from build123d import *

# Parameters (mm, degrees)
F0_W     = 210
F0_H     = 60
F1_DEPTH = 90
F2_T     = -2.5
F3_W     = 210
F3_H     = 60
F3_W_2   = 205
F3_H_2   = 55
F4_DEPTH = 2.5
F5_W     = 60
F5_H     = 50
F6_DEPTH = 25


with BuildPart() as f1:
    # F0 (on Top) → F1 (new body)
    with BuildSketch(Plane.XY):
        with Locations((2.4435054511, -41.2361205323)):
            Rectangle(F0_W, F0_H)
    extrude(amount=F1_DEPTH)

    # F2
    f2_openings = [f1.faces().sort_by_distance(p)[0] for p in [
        (2.443505, -41.236121, 90),
    ]]
    offset(amount=F2_T, openings=f2_openings)

    # F3 (on face) → F4 (join)
    with BuildSketch(Plane.XY.offset(90)):
        with Locations((2.4435054511, -41.2361205323)):
            Rectangle(F3_W, F3_H)
        with Locations((2.4435054511, -41.2361205323)):
            Rectangle(F3_W_2, F3_H_2, mode=Mode.SUBTRACT)
        with Locations((2.4435054511, -41.2361205323)):
            Rectangle(F3_W_2, F3_H_2)
    extrude(amount=F4_DEPTH)

    # F5 (on face) → F6 (cut)
    with BuildSketch(Plane.XZ.offset(71.2361205323)):
        with Locations((2.4435054511, 45)):
            Rectangle(F5_W, F5_H)
    extrude(amount=-F6_DEPTH, mode=Mode.SUBTRACT)


solid = f1.part
Could you check a few things on this model? Use its own coordinates, in mm. A direction names the side the tool comes from. Coordinates: 2 decimals unless noted, no trailing zeros. Loops run counter-clockwise (first coordinate to the right, second up) from the corner with the lowest first, then second, coordinate; pieces in that order, holes last. Notation, with made-up numbers: (-4.75, 38.5) -> (50.25, 38.5) arc R20 ccw to (50.25, 69.5) -> close; hole circle Ø9 at (76.5, -14). An arc over 180 degrees is marked (long way). Answer in a Markdown table with one row per item.
(1) If I drill on probe 1 along Y at (x, z) = (-57, 87.5); probe 2 along Z at (x, y) = (-12.5, -41); probe 3 along X at (y, z) = (-59, 48), over which ranges is the centre line in solid material (lowest first)?
Results found:
| item | result |
|---|---|
| probe 1 | y = -71.24 to -68.74, -13.74 to -11.24 |
| probe 2 | z = 0 to 2.5, 90 to 92.5 |
| probe 3 | x = -102.56 to -100.06, 104.94 to 107.44 |
(2) Thinking about a two-plate mould opening in Z: for faces 3 (the face through (1, -41, 92.5)), 4 (the face through (-102.556, -42, 46)), 5 (the face through (1, -68.736, 16)), which applies, released by +Z, released by -Z, zero draft, split by the parting line, or undercut?
Results found:
| item | result |
|---|---|
| face 3 | released by +Z |
| face 4 | zero draft |
| face 5 | undercut |
(3) For faces 1 (the face through (107.444, -42, 46)), 2 (the face through (1, -41, 2.5)), which set-ups out of +Z, -Z, +X, -X, +Y, -Y let a thin tool reach every point of the face, with its end or its side?
Results found:
| item | result |
|---|---|
| face 1 | +Z, -Z, +X, +Y, -Y |
| face 2 | none |
(4) Imagine slicing it at D-D (x = -11.5). List the corners of the cut face in (y, z) for me.
Results found:
| item | result |
|---|---|
| outline | (-71.24, 0) -> (-11.24, 0) -> (-11.24, 92.5) -> (-71.24, 92.5) -> (-71.24, 70) -> (-68.74, 70) -> (-68.74, 90) -> (-13.74, 90) -> (-13.74, 2.5) -> (-68.74, 2.5) -> (-68.74, 20) -> (-71.24, 20) -> close |
(5) Imagine slicing it at A-A (z = 87.5). List the corners of the cut face in (x, y) for me.
Results found:
| item | result |
|---|---|
| outline | (-102.56, -71.24) -> (107.44, -71.24) -> (107.44, -11.24) -> (-102.56, -11.24) -> close; hole (-100.06, -68.74) -> (104.94, -68.74) -> (104.94, -13.74) -> (-100.06, -13.74) -> close |
(6) Imagine slicing it at B-B (x = 70). List the corners of the cut face in (y, z) for me, plus the area to 4 significant figures.
Results found:
| item | result |
|---|---|
| outline | (-71.24, 0) -> (-11.24, 0) -> (-11.24, 92.5) -> (-71.24, 92.5) -> close; hole (-68.74, 2.5) -> (-13.74, 2.5) -> (-13.74, 90) -> (-68.74, 90) -> close |
| area | 737.5 mm^2 |
(7) Imagine slicing it at C-C (z = 39.5). List the corners of the cut face in (x, y) for me, plus the area to 4 significant figures.
Results found:
| item | result |
|---|---|
| outline | (-102.56, -71.24) -> (-27.56, -71.24) -> (-27.56, -68.74) -> (-100.06, -68.74) -> (-100.06, -13.74) -> (104.94, -13.74) -> (104.94, -68.74) -> (32.44, -68.74) -> (32.44, -71.24) -> (107.44, -71.24) -> (107.44, -11.24) -> (-102.56, -11.24) -> close |
| area | 1,175 mm^2 |
